```python
from build123d import *

# Parameters (mm, degrees)
SKETCH1_R            = 3.25
BOSS_EXTRUDE1_DEPTH  = 8.5
SKETCH3_W            = 65
SKETCH3_H            = 51.25
BOSS_EXTRUDE2_DEPTH  = 2.5
SKETCH4_W            = 7.6
SKETCH4_H            = 30.6
BOSS_EXTRUDE3_DEPTH  = 14
SKETCH5_R            = 3.25
BOSS_EXTRUDE4_DEPTH  = 8.5
SKETCH6_W            = 25.75
SKETCH6_H            = 2.5
BOSS_EXTRUDE5_DEPTH  = 12.25
SKETCH8_R            = 3.25
BOSS_EXTRUDE9_DEPTH  = 8.5
SKETCH9_W            = 20.5
SKETCH9_H            = 2.5
BOSS_EXTRUDE10_DEPTH = 12.25
SKETCH10_W           = 20.5
SKETCH10_H           = 12.25
CUT_EXTRUDE1_DEPTH   = 0.1
SKETCH12_W           = 25.75
SKETCH12_H           = 12.25
BOSS_EXTRUDE11_DEPTH = 0.1
SKETCH14_W           = 14
SKETCH14_H           = 30.6
BOSS_EXTRUDE12_DEPTH = 0.1


with BuildPart() as part:
    # Sketch1 → Boss-Extrude1 (new body)
    with BuildSketch(Plane.XY):
        with Locations((-17.5, -3)):
            Circle(SKETCH1_R)
    extrude(amount=BOSS_EXTRUDE1_DEPTH)

    # Sketch3 → Boss-Extrude2 (add)
    with BuildSketch(Plane.XY):
        Rectangle(SKETCH3_W, SKETCH3_H)
    extrude(amount=-BOSS_EXTRUDE2_DEPTH)

    # Sketch4 → Boss-Extrude3 (add)
    with BuildSketch(Plane.XY):
        with Locations((28.7, 0)):
            Rectangle(SKETCH4_W, SKETCH4_H)
    extrude(amount=BOSS_EXTRUDE3_DEPTH)

    # Sketch5 → Boss-Extrude4 (add)
    with BuildSketch(Plane.XY):
        with Locations((-10.25, 4)):
            Circle(SKETCH5_R)
    extrude(amount=BOSS_EXTRUDE4_DEPTH)

    # Sketch6 → Boss-Extrude5 (add)
    with BuildSketch(Plane.XY):
        with Locations((-1.875, 24.375)):
            Rectangle(SKETCH6_W, SKETCH6_H)
    extrude(amount=BOSS_EXTRUDE5_DEPTH)

    # Sketch8 → Boss-Extrude9 (add)
    with BuildSketch(Plane.XY):
        with Locations((-9.5, 19.87)):
            Circle(SKETCH8_R)
    extrude(amount=BOSS_EXTRUDE9_DEPTH)

    # Sketch9 → Boss-Extrude10 (add)
    with BuildSketch(Plane.XY):
        with Locations((4.25, -24.375)):
            Rectangle(SKETCH9_W, SKETCH9_H)
    extrude(amount=BOSS_EXTRUDE10_DEPTH)

    # Sketch10 → Cut-Extrude1 (cut)
    with BuildSketch(Plane.XZ.offset(25.625)):
        with Locations((4.25, 6.125)):
            Rectangle(SKETCH10_W, SKETCH10_H)
    extrude(amount=-CUT_EXTRUDE1_DEPTH, mode=Mode.SUBTRACT)

    # Sketch12 → Boss-Extrude11 (add)
    with BuildSketch(Plane(origin=(0, 25.625, 0), x_dir=(1, 0, 0), z_dir=(0, 1, 0))):
        with Locations((-1.875, -6.125)):
            Rectangle(SKETCH12_W, SKETCH12_H)
    extrude(amount=BOSS_EXTRUDE11_DEPTH)

    # Sketch14 → Boss-Extrude12 (add)
    with BuildSketch(Plane(origin=(32.5, 0, 0), x_dir=(0, 0, -1), z_dir=(1, 0, 0))):
        with Locations((-7, 0)):
            Rectangle(SKETCH14_W, SKETCH14_H)
    extrude(amount=BOSS_EXTRUDE12_DEPTH)


solid = part.part
```
Work out the finished part from the listing and answer in its coordinate system (mm). A direction names the side the tool comes from. Round coordinates to 2 decimals unless told otherwise and drop trailing zeros. Order: outer loops, then holes, each group sorted by start corner. A loop starts at its lowest first (then second) coordinate and runs counter-clockwise, first axis right, second up.
Q1. Given pin 1 Ø2 at (x, y) = (-16, -4) entering from +Z; pin 2 Ø4 at (x, z) = (27, 6.5) entering from -Y; pin 3 Ø0.8 at (x, y) = (2.5, 24.5) entering from +Z, each flat-ended and moving along its own axis, determine where each tip first touches the part or whether it passes through.
Solution:
pin 1: stops at z = 8.5
pin 2: stops at y = -15.3
pin 3: stops at z = 12.25
Q2. A cutting plane is placed at B-B, the plane x = 13.5. Determine the outline of the cut face in (y, z) (3 decimals), then the cut area to 3 significant figures.
Solution:
outline: (-25.625, -2.5) - (25.625, -2.5) - (25.625, 0) - (-23.125, 0) - (-23.125, 12.25) - (-25.525, 12.25) - (-25.525, 0) - (-25.625, 0) - close
area: 158 mm2
Q3. A cutting plane is placed at C-C, the plane y = -7.5. Determine the outline of the cut face in (x, z), then the cut area to 3 significant figures.
Solution:
outline: (-32.5, -2.5) - (32.5, -2.5) - (32.5, 0) - (32.6, 0) - (32.6, 14) - (24.9, 14) - (24.9, 0) - (-32.5, 0) - close
area: 270 mm2
Q4. A tool of negligible diameter and unlimited length cuts with its end or side. For faces 1 (the cylindrical face through (-13.5, 4.1, 4.2)), 2 (the flat face through (32.5, 0, -1)), 3 (the flat face through (-6, -24, 6)), from which of +Z, -Z, +X, -X, +Y, -Y can it reach the whole face along a straight path? Write none if from no direction.
Solution:
face 1: +Z
face 2: -Z, +X, +Y, -Y
face 3: +Z, -X, -Y
Q5. A cutting plane is placed at D-D, the plane y = -19. Determine the outline of the cut face in (x, z), then the cut area to 4 significant figures.
Solution:
outline: (-32.5, -2.5) - (32.5, -2.5) - (32.5, 0) - (-32.5, 0) - close
area: 162.5 mm2
Q6. The mould has two halves that part along Y. Classify faces 4 (the flat face through (-14.75, 24, 6)), 5 (the flat face through (4, -23.125, 6)), 6 (the flat face through (29, -15.3, 7)): pulls with the +Y half, pulls with the -Y half, needs draft (parallel to the pull), parting line crosses it, or undercut.
Solution:
face 4: needs draft
face 5: undercut
face 6: pulls with the -Y half
Q7. A cutting plane is placed at A-A, the plane z = 4. Determine the outline of the cut face in (x, y) (3 decimals), then the cut area to 3 significant figures.
Solution:
outline: circle Ø6.5 at (-17.5, -3); (-14.75, 23.125) - (11, 23.125) - (11, 25.725) - (-14.75, 25.725) - close; circle Ø6.5 at (-10.25, 4); circle Ø6.5 at (-9.5, 19.87); (-6, -25.525) - (14.5, -25.525) - (14.5, -23.125) - (-6, -23.125) - close; (24.9, -15.3) - (32.6, -15.3) - (32.6, 15.3) - (24.9, 15.3) - close
area: 451 mm2
Q8. Find the intervals of material crossed by line 1 along Y through (x, z) = (9, 5) (3 decimals); line 2 along X through (y, z) = (-4, 2); line 3 along Z through (x, y) = (-6, -11), in increasing order.
Solution:
line 1: y = -25.525 to -23.125, 23.125 to 25.725
line 2: x = -20.59 to -14.41, 24.9 to 32.6
line 3: z = -2.5 to 0
